from build123d import *

# Parameters (mm, degrees)
SKETCH_1_W          = 780
SKETCH_1_H          = 300
EXTRUDE_1_DEPTH     = 3
FILLET_3_R          = 20
CHAMFER_1_SIZE      = 0.8
SKETCH_2_R          = 3.25
CUT_EXTRUDE_1_DEPTH = 10


with BuildPart() as part:
    # 草图1 → 凸台-拉伸1 (new body)
    with BuildSketch(Plane(origin=(0, 0, 0), x_dir=(1, 0, 0), z_dir=(0, 1, 0))):
        with Locations((390, 150)):
            Rectangle(SKETCH_1_W, SKETCH_1_H)
        Polygon((600, 405), (305, 405), (230, 300), (305, 300), (600, 300), (675, 300), align=None)
    extrude(amount=EXTRUDE_1_DEPTH)

    # 圆角3
    fillet_3_edges = [part.edges().sort_by_distance(p)[0] for p in [
        (0, 1.5, 0),
        (0, 1.5, -300),
        (230, 1.5, -300),
        (305, 1.5, -405),
        (600, 1.5, -405),
        (675, 1.5, -300),
        (780, 1.5, -300),
        (780, 1.5, 0),
    ]]
    fillet(fillet_3_edges, radius=FILLET_3_R)

    # 倒角1
    chamfer_1_edges = [part.edges().sort_by_distance(p)[0] for p in [
        (390, 0, 0),
        (390, 3, 0),
        (0, 0, -150),
        (119.853821047, 0, -300),
        (267.5, 0, -352.5),
        (452.5, 0, -405),
        (637.5, 0, -352.5),
        (722.646178953, 0, -300),
        (780, 0, -150),
        (5.857864376, 0, -294.142135624),
        (774.142135624, 0, -5.857864376),
        (774.142135624, 0, -294.142135624),
        (598.859273711, 0, -402.783352854),
        (306.140726289, 0, -402.783352854),
        (5.857864376, 0, -5.857864376),
        (0, 3, -150),
        (780, 3, -150),
        (722.646178953, 3, -300),
        (637.5, 3, -352.5),
        (452.5, 3, -405),
        (267.5, 3, -352.5),
        (119.853821047, 3, -300),
        (5.857864376, 3, -294.142135624),
        (774.142135624, 3, -5.857864376),
        (774.142135624, 3, -294.142135624),
        (598.859273711, 3, -402.783352854),
        (306.140726289, 3, -402.783352854),
        (5.857864376, 3, -5.857864376),
        (228.859273711, 0, -302.216647146),
        (228.859273711, 3, -302.216647146),
        (676.140726289, 0, -302.216647146),
        (676.140726289, 3, -302.216647146),
    ]]
    chamfer(chamfer_1_edges, length=CHAMFER_1_SIZE)

    # 草图2 → 切除-拉伸1 (cut)
    with BuildSketch(Plane(origin=(0, 3, 0), x_dir=(1, 0, 0), z_dir=(0, 1, 0))):
        with Locations(Location((70.8, 170.8, 0), (0, 0, 270))):
            Circle(SKETCH_2_R)
        with Locations(Location((749.2, 269.2, 0), (0, 0, 270))):
            Circle(SKETCH_2_R)
        with Locations(Location((749.2, 30.8, 0), (0, 0, 270))):
            Circle(SKETCH_2_R)
        with Locations(Location((155.8, 30.8, 0), (0, 0, 270))):
            Circle(SKETCH_2_R)
        with Locations(Location((155.8, 269.2, 0), (0, 0, 270))):
            Circle(SKETCH_2_R)
    extrude(amount=-CUT_EXTRUDE_1_DEPTH, mode=Mode.SUBTRACT)


solid = part.part
Here's how the part is built. I have some questions about the finished solid (model axes, mm). Round coordinates to 2 decimals unless told otherwise and drop trailing zeros. Order: outer loops, then holes, each group sorted by start corner. A loop starts at its lowest first (then second) coordinate and runs counter-clockwise, first axis right, second up. Notation, with made-up numbers: (51, -30) -> (81, -30) arc R23 ccw to (81, -13) -> close; hole circle Ø2 at (11.25, -24.5). An arc over 180 degrees is marked (long way). Use CSV: the item, a comma, the result in double quotes.
1. I want a section at B-B on x = 110. List the corners of the cut face in (y, z) for me, and give its area (3 significant figures).
Recorded:
outline,"(0, -299.2) -> (0.8, -300) -> (2.2, -300) -> (3, -299.2) -> (3, -0.8) -> (2.2, 0) -> (0.8, 0) -> (0, -0.8) -> close"
area,"899 mm2"
2. I need wall thicknesses on line 1 along Z through (x, y) = (155.8, 2.05); line 2 along X through (y, z) = (1.5, -269.2); line 3 along Z through (x, y) = (204.5, 1.9). Which ranges of each line are inside material? Lowest first, please.
Recorded:
line 1,"z = -300 to -272.45, -265.95 to -34.05, -27.55 to 0"
line 2,"x = 0 to 152.55, 159.05 to 745.95, 752.45 to 780"
line 3,"z = -300 to 0"
3. I want a section at A-A on y = 1.6. List the corners of the cut face in (x, z) for me, and give its area (3 significant figures).
Recorded:
outline,"(0, -280) arc R20 ccw to (20, -300) -> (219.71, -300) arc R20 cw to (235.98, -308.38) -> (299.02, -396.62) arc R20 ccw to (315.29, -405) -> (589.71, -405) arc R20 ccw to (605.98, -396.62) -> (669.02, -308.38) arc R20 cw to (685.29, -300) -> (760, -300) arc R20 ccw to (780, -280) -> (780, -20) arc R20 ccw to (760, 0) -> (20, 0) arc R20 ccw to (0, -20) -> close; hole circle Ø6.5 at (70.8, -170.8); hole circle Ø6.5 at (155.8, -269.2); hole circle Ø6.5 at (155.8, -30.8); hole circle Ø6.5 at (749.2, -269.2); hole circle Ø6.5 at (749.2, -30.8)"
area,"272,000 mm2"
